Autodesk Inventor part; units mm, degrees
ref_plane "Work Plane1" through (0, 0, 0) normal (0, -0.7071068, 0.7071068) x (1, 0, 0)
ref_plane "YZ Plane" through (0, 0, 0) normal (1, 0, 0) x (0, 1, 0)
ref_plane "XZ Plane" through (0, 0, 0) normal (0, 1, 0) x (-1, 0, 0)
sketch "Sketch1" plane through (0, 0, 0) normal (0, 0, 1) x (1, 0, 0)
  circle A0 centre (0, 0) radius 100 construction
  circle A1 centre (0, 0) radius 75 construction
  circle A2 centre (0, 75) radius 25 construction
  circle A3 centre (0, 0) radius 89 construction
  dimension "d1" = 150
  dimension "d0" = 200
  dimension "d3" = 50
  dimension "d4" = 14
ref_plane "Work Plane1" through (0, 0, 0) normal (0, -0.7071068, 0.7071068) x (1, 0, 0)
sketch "Sketch2" plane through (0, 0, 0) normal (0, -0.7071068, 0.7071068) x (1, 0, 0)
  ellipse E0 centre (0, 0) end of major axis (100, 0) minor radius 70.7107 construction
  circle A0 centre (0, 45.7107) radius 25 construction
  circle A1 centre (0, 45.7107) radius 22 construction
  circle A2 centre (0, 45.7107) radius 12.5 construction
  line L0 (0, 58.2107) -> (46.793, 58.2107) construction
  line L1 (46.793, 45.7107) -> (-46.793, 45.7107)
  line L2 (0, 45.7107) -> (0, 58.2107) construction
  line L3 (0, 58.2107) -> (-46.793, 58.2107) construction
  ellipse E1 centre (0, 0) end of major axis (-96.8498, 0) minor radius 67.7107 (49.4713, 58.2107) -> (-49.4713, 58.2107) ccw construction
  line L4 (-46.793, 58.2107) -> (-46.793, 45.7107)
  line L5 (46.793, 58.2107) -> (46.793, 45.7107)
  circle A3 centre (0, 45.7107) radius 21 construction
  spline S0 degree 5 poles (103, 0) (102.9997, 6.0067) (102.15, 12.0166) (100.4439, 17.8567) (95.335, 29.4916) (87.5543, 39.5637) (82.9111, 44.3403) (72.1684, 53.435) (59.9286, 60.4121) (53.1788, 63.5338) (38.7726, 68.8984) (23.7279, 72.0795) (15.8518, 73.167) (0.0001, 74.2544) (-15.8515, 73.167) (-23.7275, 72.0796) (-38.7724, 68.8985) (-53.1787, 63.534) (-59.9287, 60.4119) (-72.1688, 53.435) (-82.9115, 44.3398) (-87.5547, 39.5637) (-95.3351, 29.4907) (-100.4441, 17.8572) (-102.1497, 12.015) (-103.8502, 0) (-102.1497, -12.015) (-100.4441, -17.8572) (-95.3351, -29.4907) (-87.5547, -39.5637) (-82.9115, -44.3398) (-72.1688, -53.435) (-59.9287, -60.4119) (-53.1787, -63.534) (-38.7724, -68.8985) (-23.7275, -72.0796) (-15.8515, -73.167) (0.0001, -74.2544) (15.8518, -73.167) (23.7279, -72.0795) (38.7726, -68.8984) (53.1788, -63.5338) (59.9286, -60.4121) (72.1684, -53.435) (82.9111, -44.3403) (87.5543, -39.5637) (95.335, -29.4916) (100.4439, -17.8567) (102.15, -12.0166) (102.9997, -6.0067) (103, 0) knots 0 0 0 0 0 0 0.053721 0.053721 0.053721 0.112881 0.112881 0.112881 0.179119 0.179119 0.179119 0.25 0.25 0.25 0.320879 0.320879 0.320879 0.38712 0.38712 0.38712 0.44628 0.44628 0.44628 0.5 0.5 0.5 0.55372 0.55372 0.55372 0.61288 0.61288 0.61288 0.679121 0.679121 0.679121 0.75 0.75 0.75 0.820881 0.820881 0.820881 0.887119 0.887119 0.887119 0.946279 0.946279 0.946279 1 1 1 1 1 1 construction
  spline S1 degree 5 poles (125, 0) (124.9996, 8.8962) (123.6824, 17.7961) (121.0383, 26.425) (113.3824, 42.8537) (101.833, 56.8343) (95.2127, 63.1614) (80.4494, 74.6213) (63.7738, 83.0792) (54.8985, 86.6443) (36.372, 92.4116) (17.1764, 95.263) (7.3437, 95.9828) (-12.2502, 95.9826) (-31.6302, 93.1025) (-41.1422, 90.9507) (-59.3601, 85.2856) (-76.3656, 76.6479) (-84.2872, 71.6905) (-98.7984, 60.4396) (-110.4889, 46.2955) (-115.3769, 38.6773) (-122.9533, 22.3258) (-125.6666, 4.5154) (-125.6666, -4.5154) (-122.9533, -22.3258) (-115.3769, -38.6773) (-110.4889, -46.2955) (-98.7984, -60.4396) (-84.2872, -71.6905) (-76.3656, -76.6479) (-59.3601, -85.2856) (-41.1422, -90.9507) (-31.6302, -93.1025) (-12.2502, -95.9826) (7.3437, -95.9828) (17.1764, -95.263) (36.372, -92.4116) (54.8985, -86.6443) (63.7738, -83.0792) (80.4494, -74.6213) (95.2127, -63.1614) (101.833, -56.8343) (113.3824, -42.8537) (121.0383, -26.425) (123.6824, -17.7961) (124.9996, -8.8962) (125, 0) knots 0 0 0 0 0 0 0.063791 0.063791 0.063791 0.128941 0.128941 0.128941 0.197218 0.197218 0.197218 0.267663 0.267663 0.267663 0.337325 0.337325 0.337325 0.403955 0.403955 0.403955 0.468142 0.468142 0.468142 0.531858 0.531858 0.531858 0.596045 0.596045 0.596045 0.662675 0.662675 0.662675 0.732337 0.732337 0.732337 0.802782 0.802782 0.802782 0.871059 0.871059 0.871059 0.936209 0.936209 0.936209 1 1 1 1 1 1 construction
  spline S2 degree 5 poles (46.793, 58.2107) (42.0231, 60.0696) (37.1481, 61.6587) (32.1958, 62.9892) (18.4817, 65.9465) (4.4646, 67.0684) (-4.4646, 67.0684) (-18.4817, 65.9465) (-32.1958, 62.9892) (-37.1481, 61.6587) (-42.0231, 60.0696) (-46.793, 58.2107) knots 0 0 0 0 0 0 0.267579 0.267579 0.267579 0.732421 0.732421 0.732421 1 1 1 1 1 1
  point P0 (0, 53.033)
  point P1 (0, 53.033)
  dimension "d17" = 3
  dimension "d28" = 25
  dimension "d25" = 50
  dimension "d27" = 3
  dimension "d29" = 9.5
  dimension "d50" = 46.793
  dimension "d51" = 46.793
  dimension "d52" = 1
revolve "Revolution1" add sketch "Sketch2" angle 360 about axis through (46.793, 32.3223, 32.3223) along (-1, 0, 0)
sketch "Sketch5" plane through (-46.793, 32.3223, 32.3223) normal (-1, 0, 0) x (0, 0, 1)
  circle A0 centre (0, 0) radius 12.5
  circle A1 centre (0, 0) radius 11
  point P0 (-32.3223, -32.3223)
  point P1 (8.8388, 8.8388)
  dimension "d53" = 22
extrude "Extrusion3" cut sketch "Sketch5" against normal blind 7 contours A1
sketch "Sketch6" plane through (46.793, 32.3223, 32.3223) normal (1, 0, 0) x (0, 0, -1)
  circle A0 centre (0, 0) radius 12.5
  circle A1 centre (0, 0) radius 11
  point P0 (32.3223, -32.3223)
  point P1 (-8.8388, 8.8388)
  dimension "d56" = 22
extrude "Extrusion4" cut sketch "Sketch6" against normal blind 7 contours A1
hole "Hole2" at (-39.793, 32.3223, 32.3223) direction (1, 0, 0) diameter 16 end up to surface
properties part number "Roller 48mm"
CAD build for the part. Positions are in the model's coordinates, mm. A direction names the side the tool comes from. Give positions to 0.01 mm unless a question says otherwise; leave off trailing zeros. Write each question's results on one line, items separated by ' | '.
1. Wall check: probe 1 along X at (y, z) = (26, 24); probe 2 along Z at (x, y) = (3, 35.5); probe 3 along Y at (x, z) = (-16.5, 30). Give the ranges that are in metal, low to high. Write a range as [from, to].
Geometry check:
probe 1: [-39.79, 39.79] | probe 2: [11.6, 24.98], [39.66, 53.05] | probe 3: [12.45, 24.67], [39.98, 52.19]
2. Two-plate mould, pull along Z, no slides. Class faces 4 (the flat face through (46.793, 24, 40)), 5 (the flat face through (39.793, 24, 32)): pulls with the +Z half, pulls with the -Z half, needs draft (parallel to the pull), parting line crosses it, or undercut.
Geometry check:
face 4: needs draft | face 5: undercut
3. Which spindle directions (+Z, -Z, +X, -X, +Y, -Y) get a long thin tool onto all of the face, cutting with end or side? Do faces 1 (the flat face through (-46.793, 24, 40)), 2 (the cylindrical face through (43.34, 25.63, 41.05)), 3 (the flat face through (-39.793, 24, 33)). Say none if no direction does.
Geometry check:
face 1: +Z, -Z, -X, +Y, -Y | face 2: +X | face 3: -X
4. Drop flat-ended pins along their axis: P1, Ø8, axis at x = 21, y = 37, coming from the -Z side; P2, Ø5, axis at x = 4.5, z = 21.5, coming from the +Y side; P3, Ø1.5, axis at x = 12.5, y = 47, coming from the +Z side. Give the stop position or say it passes through.
Geometry check:
P1: z = 12.61 | P2: y = 51.53 | P3: z = 47.27
